Part model, mm, in its own coordinate system. A direction names the side the tool comes from. Coordinates: 2 decimals unless noted, no trailing zeros. Loops run counter-clockwise (first coordinate to the right, second up) from the corner with the lowest first, then second, coordinate; pieces in that order, holes last. Notation, with made-up numbers: (35, 87) -> (57, 87) arc R20 cw to (57, 92) -> close; hole circle Ø4 at (67.5, 87). An arc over 180 degrees is marked (long way). Use one line per item in the form item = value. Start each with the question number.
(1) Mould opens along Z. For faces 1 (the cylindrical face through (1.907, 12.522, -6.643)), 2 (the flat face through (182, 25.4, -13)), 3 (the flat face through (287, 14, -25.4)) say: +Z half, -Z half, draft (parallel to the pull), parting line (faces both ways), or undercut.
(2) Pin check, flat tips, straight feed: P1, Ø11.5, axis at x = 565.15, z = -12.7, coming from the -Y side; P2, Ø2, axis at x = 333.5, z = -12, coming from the +Y side; P3, Ø3, axis at y = 39, z = -12, coming from the -X side; P4, Ø7.5, axis at y = 35.5, z = -8, coming from the +X side. Stop position of each tip, or through.
(3) Band-saw the part on B-B on y = 13.5. Give the cut face in (x, z) (3 decimals), then the cut area to 3 significant figures.
(4) 3-axis set-ups, long thin cutter, end or side, ignore diameter. For faces 4 (the flat face through (412.75, 38, -13)), 5 (the flat face through (374.65, 38, -13)), 6 (the flat face through (393, 51.943, -13)): which of +Z, -Z, +X, -X, +Y, -Y reach the whole face in a straight line?
(5) Band-saw the part on C-C on x = 107. Give the cut face in (y, z).
(6) Band-saw the part on A-A on y = 39.5. Give the cut face in (x, z) (3 decimals), then the cut area to 3 significant figures.
(7) Drill centre lines: L1, parallel to X at y = 7, z = -12.7 (3 decimals); L2, parallel to X at y = 20, z = -8.75; L3, parallel to X at y = 9, z = -10.5. Where is each one in solid material? Low to high. Write a range as [from, to].
```python
from build123d import *

# Parameters (mm, degrees)
SKETCH2_R           = 6.35
SKETCH2_R_2         = 3.175
BOSS_EXTRUDE1_DEPTH = 25.4
SKETCH14_W          = 38.1
SKETCH14_H          = 25.4
BOSS_EXTRUDE2_DEPTH = 26.543
SKETCH15_R          = 3.175
CUT_EXTRUDE1_DEPTH  = 19.05
FILLET1_R           = 7.62


with BuildPart() as part:
    # Sketch2 → Boss-Extrude1 (new body)
    with BuildSketch(Plane(origin=(0, 0, 0), x_dir=(1, 0, 0), z_dir=(0, 1, 0))):
        with BuildLine():
            ThreePointArc((0, 25.4), (-12.7, 12.7), (0, 0))
            Line((0, 0), (565.15, 0))
            ThreePointArc((565.15, 0), (577.85, 12.7), (565.15, 25.4))
            Line((565.15, 25.4), (0, 25.4))
        make_face()
        with Locations(Location((0, 12.7, 0), (0, 0, 270))):
            Circle(SKETCH2_R, mode=Mode.SUBTRACT)
        with Locations(Location((120.65, 12.7, 0), (0, 0, 270))):
            Circle(SKETCH2_R_2, mode=Mode.SUBTRACT)
        with Locations(Location((565.15, 12.7, 0), (0, 0, 270))):
            Circle(SKETCH2_R, mode=Mode.SUBTRACT)
    extrude(amount=BOSS_EXTRUDE1_DEPTH)

    # Sketch14 → Boss-Extrude2 (add)
    with BuildSketch(Plane(origin=(0, 25.4, 0), x_dir=(1, 0, 0), z_dir=(0, 1, 0))):
        with Locations((393.7, 12.7)):
            Rectangle(SKETCH14_W, SKETCH14_H)
    extrude(amount=BOSS_EXTRUDE2_DEPTH)

    # Sketch15 → Cut-Extrude1 (cut)
    with BuildSketch(Plane(origin=(0, 51.943, 0), x_dir=(1, 0, 0), z_dir=(0, 1, 0))):
        with Locations(Location((381, 12.7, 0), (0, 0, 270))):
            Circle(SKETCH15_R)
    extrude(amount=-CUT_EXTRUDE1_DEPTH, mode=Mode.SUBTRACT)

    # Fillet1
    fillet1_edges = [part.edges().sort_by_distance(p)[0] for p in [
        (374.65, 38.6715, 0),
        (374.65, 38.6715, -25.4),
    ]]
    fillet(fillet1_edges, radius=FILLET1_R)


solid = part.part
```
A:
q1.face_1 = undercut
q1.face_2 = draft
q1.face_3 = -Z half
q2.P1 = through
q2.P2 = 25.4
q2.P3 = 374.65
q2.P4 = 412.75
q3.outline = (0, -25.4) -> (565.15, -25.4) arc R12.7 ccw to (565.15, 0) -> (0, 0) arc R12.7 ccw to start; hole circle Ø12.7 at (0, -12.7); hole circle Ø6.35 at (120.65, -12.7); hole circle Ø12.7 at (565.15, -12.7)
q3.area = 14,600 mm²
q4.face_4 = +Z, -Z, +X, +Y
q4.face_5 = +Z, -Z, -X, +Y
q4.face_6 = +Z, -Z, +X, -X, +Y
q5.outline = (0, -25.4) -> (25.4, -25.4) -> (25.4, 0) -> (0, 0) -> close
q6.outline = (374.65, -17.78) arc R7.62 ccw to (382.27, -25.4) -> (412.75, -25.4) -> (412.75, 0) -> (382.27, 0) arc R7.62 ccw to (374.65, -7.62) -> close; hole circle Ø6.35 at (381, -12.7)
q6.area = 911 mm²
q7.L1 = [-12.7, -6.35], [6.35, 117.475], [123.825, 558.8], [571.5, 577.85]
q7.L2 = [-12.07, -4.97], [4.97, 560.18], [570.12, 577.22]
q7.L3 = [-12.51, -5.96], [5.96, 118.36], [122.94, 559.19], [571.11, 577.66]
